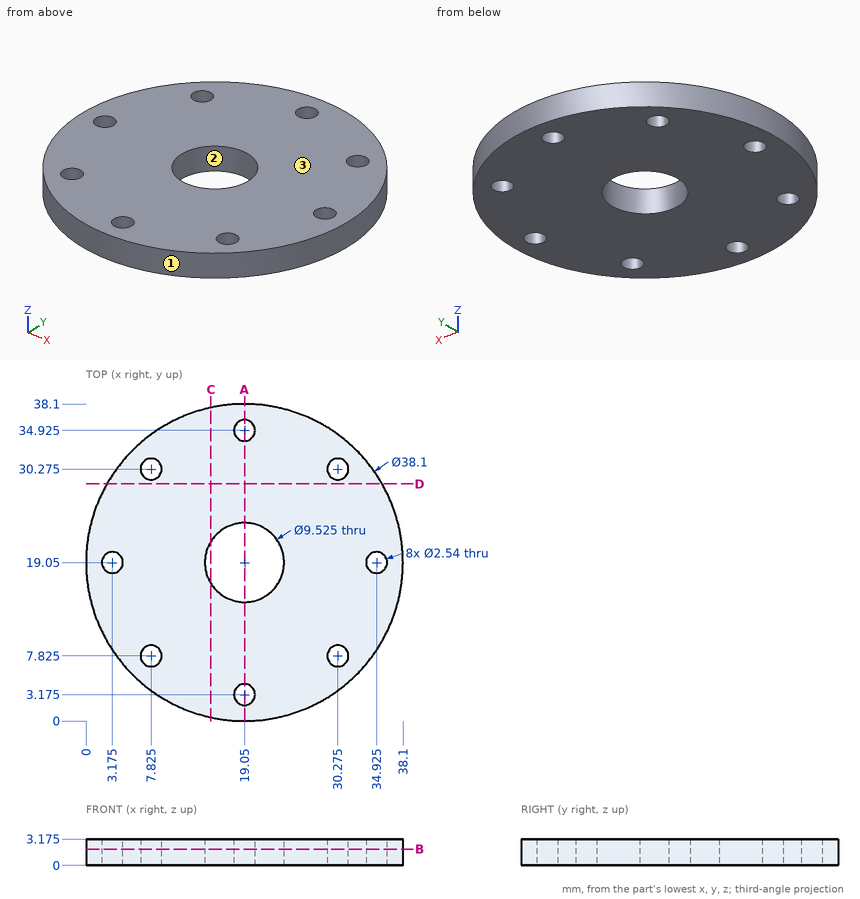
Study the drawing (mm; zero at the part's minimum x, y, z) and answer. Round coordinates to 2 decimals unless told otherwise and drop trailing zeros. Loops run counter-clockwise (first coordinate to the right, second up) from the corner with the lowest first, then second, coordinate; pieces in that order, holes last.
Q1. Section C-C, the plane x = 15 is taken. Determine the outline of the cut face in (y, z) (1 decimal), then the cut area to 3 significant figures.
Q2. Given pin 1 Ø3.5 at (x, y) = (3.175, 19.05) entering from +Z (3 decimals); pin 2 Ø1.5 at (x, z) = (14.5, 0.5) entering from +Y, each flat-ended and moving along its own axis, determine where each tip first touches the part or whether it passes through.
Q3. Section B-B, the plane z = 1.95 is taken. Count the separate pieces of the cut face and the enclosed holes in it, then the cut area to 3 significant figures.
Q4. Find the intervals of material crossed by line 1 (Y direction, x = 19.05, z = 2.1) (1 decimal); line 2 (Y direction, x = 34, z = 1.2) (1 decimal); line 3 (Y direction, x = 15, z = 0.65) (1 decimal), in increasing order.
Q5. For a pull along X with two mould halves and no side action, classify the marked faces 1, 2 and 3 as released by +X, released by -X, zero draft, split by the parting line, or undercut.
Q6. Section D-D, the plane y = 28.5 is taken. Determine the outline of the cut face in (x, z) (1 decimal).
Q7. Section A-A, the plane x = 19.05 is taken. Determine the outline of the cut face in (y, z) (1 decimal), then the cut area to 3 significant figures.
Completed:
1. outline: (0.4, 0) - (16.5, 0) - (16.5, 3.2) - (0.4, 3.2) - close; (21.6, 0) - (37.7, 0) - (37.7, 3.2) - (21.6, 3.2) - close
1. area: 102 mm2
2. pin 1: stops at z = 3.175
2. pin 2: stops at y = 37.72
3. separate pieces: 1
3. enclosed holes: 9
3. area: 1,030 mm2
4. line 1: y = 0 to 1.9, 4.4 to 14.3, 23.8 to 33.7, 36.2 to 38.1
4. line 2: y = 7.2 to 18.2, 19.9 to 30.9
4. line 3: y = 0.4 to 16.5, 21.6 to 37.7
5. face 1: split by the parting line
5. face 2: undercut
5. face 3: zero draft
6. outline: (2.5, 0) - (35.6, 0) - (35.6, 3.2) - (2.5, 3.2) - close
7. outline: (0, 0) - (1.9, 0) - (1.9, 3.2) - (0, 3.2) - close; (4.4, 0) - (14.3, 0) - (14.3, 3.2) - (4.4, 3.2) - close; (23.8, 0) - (33.7, 0) - (33.7, 3.2) - (23.8, 3.2) - close; (36.2, 0) - (38.1, 0) - (38.1, 3.2) - (36.2, 3.2) - close
7. area: 74.6 mm2
